Model file for the job. Use its own axes, mm. A direction names the side the tool comes from. Coordinates: 2 decimals unless noted, no trailing zeros. Write each loop counter-clockwise with the first axis right and the second up, starting at its lowest first coordinate (ties: lowest second). Pieces come first, ordered by that corner, then holes. Notation, with made-up numbers: (40, 17.5) - (70, 17.5) arc R32 ccw to (70, 45.5) - close; hole circle Ø9 at (72.5, 7.5). An arc over 180 degrees is marked (long way). Put each result on its own line as item: value. Start each with the question number.
1. Pull direction Y, two halves, no side cores. Call faces 1 (the face through (24, -20.599, 2)), 2 (the face through (-26, -1.549, 2)), 3 (the face through (100.072, 31.851, 1.571)): released by +Y, released by -Y, zero draft, split by the parting line, or undercut.
2. Drop a flat-ended pin along its axis: P1, Ø1.5, axis at y = -0.5, z = 1.5, coming from the -X side. Give the stop position or say it passes through.
3. Drill centre lines: L1, parallel to Y at x = 76.2, z = 2; L2, parallel to Y at x = -2, z = 2.6; L3, parallel to X at y = -18, z = 0.85. Where is each one in solid material? Low to high. Write a range as from..to.
4. Saw through at B-B, the plane z = 1.15. Write the cut outline in (x, y), plus the area to 3 significant figures.
5. Which spindle directions (+Z, -Z, +X, -X, +Y, -Y) get a long thin tool onto all of the face, cutting with end or side? Do faces 4 (the face through (-50.8, 15, 2)), 5 (the face through (0, 0, 2)). Say none if no direction does.
6. Saw through at A-A, the plane x = -8. Write the cut outline in (y, z), plus the area to 3 significant figures.
```python
from build123d import *

# Parameters (mm, degrees)
BOSS_EXTRUDE1_DEPTH = 3.0988
SKETCH3_R           = 1.0795
BOSS_EXTRUDE2_DEPTH = 3.0988
FILLET1_R           = 5.08


with BuildPart() as part:
    # Sketch2 → Boss-Extrude1 (new body)
    with BuildSketch(Plane.XY):
        Polygon((-50.8, 1.5494), (-50.8, 7.8994), (50.8, 7.8994), (50.8, -7.8994), (-50.8, -7.8994), (-50.8, -1.5494), (0, -1.5494), (0, 1.5494), align=None)
    extrude(amount=BOSS_EXTRUDE1_DEPTH)

    # Sketch3 → Boss-Extrude2 (add)
    with BuildSketch(Plane.XY):
        Polygon((50.8, -7.8994), (-50.8, -7.8994), (-50.8, -20.5994), (101.6, -20.5994), (101.6, 33.2994), (-50.8, 33.2994), (-50.8, 7.8994), (50.8, 7.8994), align=None)
        with Locations((76.2, 0)):
            Circle(SKETCH3_R, mode=Mode.SUBTRACT)
    extrude(amount=BOSS_EXTRUDE2_DEPTH)

    # Fillet1
    fillet1_edges = [part.edges().sort_by_distance(p)[0] for p in [
        (101.6, -20.5994, 1.5494),
        (101.6, 33.2994, 1.5494),
        (-50.8, 33.2994, 1.5494),
        (-50.8, -20.5994, 1.5494),
    ]]
    fillet(fillet1_edges, radius=FILLET1_R)


solid = part.part
```
Final values:
1. face 1: released by -Y
1. face 2: undercut
1. face 3: released by +Y
2. P1: stops at x = 0
3. L1: y = -20.6..-1.08, 1.08..33.3
3. L2: y = -20.6..-1.55, 1.55..33.3
3. L3: x = -50.15..100.95
4. outline: (-50.8, -15.52) arc R5.08 ccw to (-45.72, -20.6) - (96.52, -20.6) arc R5.08 ccw to (101.6, -15.52) - (101.6, 28.22) arc R5.08 ccw to (96.52, 33.3) - (-45.72, 33.3) arc R5.08 ccw to (-50.8, 28.22) - (-50.8, 1.55) - (0, 1.55) - (0, -1.55) - (-50.8, -1.55) - close; hole circle Ø2.16 at (76.2, 0)
4. area: 8,030 mm²
5. face 4: +Z, -Z, -X, +Y, -Y
5. face 5: +Z, -Z, -X
6. outline: (-20.6, 0) - (-1.55, 0) - (-1.55, 3.1) - (-20.6, 3.1) - close; (1.55, 0) - (33.3, 0) - (33.3, 3.1) - (1.55, 3.1) - close
6. area: 157 mm²
